from build123d import *

# Parameters (mm, degrees)
CROQUIS1_W              = 76
CROQUIS1_H              = 85
SALIENTE_EXTRUIR1_DEPTH = 5
SALIENTE_EXTRUIR5_DEPTH = 5
CROQUIS6_W              = 76
CROQUIS6_H              = 85
CROQUIS6_W_2            = 68
CROQUIS6_H_2            = 77
SALIENTE_EXTRUIR6_DEPTH = 50
REDONDEO1_R             = 10
CROQUIS7_W              = 15
CROQUIS7_H              = 28
CORTAR_EXTRUIR2_DEPTH   = 5
CROQUIS8_W              = 30
CROQUIS8_H              = 30
CORTAR_EXTRUIR3_DEPTH   = 3
CROQUIS10_W             = 4
CROQUIS10_H             = 4
SALIENTE_EXTRUIR7_DEPTH = 1.5


with BuildPart() as part:
    # Croquis1 → Saliente-Extruir1 (new body)
    with BuildSketch(Plane.XY):
        Rectangle(CROQUIS1_W, CROQUIS1_H)
    extrude(amount=SALIENTE_EXTRUIR1_DEPTH)

    # Croquis5 → Saliente-Extruir5 (add)
    with BuildSketch(Plane.XY.offset(5)):
        Polygon((25.754700538, -30), (22, -30), (22, -34), (34, -34), (34, -22), (30, -22), (30, -25.575128869), (31.4, -28), (29.7, -30.944486373), (26.3, -30.944486373), align=None)
        Polygon((22, -22), (22, -30), (25.754700538, -30), (24.6, -28), (26.3, -25.055513627), (29.7, -25.055513627), (30, -25.575128869), (30, -22), align=None)
        Polygon((-22, -30), (-25.754700538, -30), (-26.3, -30.944486373), (-29.7, -30.944486373), (-31.4, -28), (-30, -25.575128869), (-30, -22), (-34, -22), (-34, -34), (-22, -34), align=None)
        Polygon((-24.6, -28), (-25.754700538, -30), (-22, -30), (-22, -22), (-30, -22), (-30, -25.575128869), (-29.7, -25.055513627), (-26.3, -25.055513627), align=None)
        Polygon((-30, 25.575128869), (-30, 22), (-22, 22), (-22, 30), (-25.754700538, 30), (-24.6, 28), (-26.3, 25.055513627), (-29.7, 25.055513627), align=None)
        Polygon((-34, 22), (-30, 22), (-30, 25.575128869), (-31.4, 28), (-29.7, 30.944486373), (-26.3, 30.944486373), (-25.754700538, 30), (-22, 30), (-22, 34), (-34, 34), align=None)
        Polygon((30, 25.575128869), (30, 22), (34, 22), (34, 34), (22, 34), (22, 30), (25.754700538, 30), (26.3, 30.944486373), (29.7, 30.944486373), (31.4, 28), align=None)
        Polygon((22, 22), (30, 22), (30, 25.575128869), (29.7, 25.055513627), (26.3, 25.055513627), (24.6, 28), (25.754700538, 30), (22, 30), align=None)
    extrude(amount=SALIENTE_EXTRUIR5_DEPTH)

    # Croquis6 → Saliente-Extruir6 (add)
    with BuildSketch(Plane.XY.offset(5)):
        Rectangle(CROQUIS6_W, CROQUIS6_H)
        Rectangle(CROQUIS6_W_2, CROQUIS6_H_2, mode=Mode.SUBTRACT)
    extrude(amount=SALIENTE_EXTRUIR6_DEPTH)

    # Redondeo1
    redondeo1_edges = [part.edges().sort_by_distance(p)[0] for p in [
        (0, 42.5, 0),
        (38, 0, 0),
        (0, -42.5, 0),
        (-38, 0, 0),
        (-38, 42.5, 27.5),
        (38, 42.5, 27.5),
        (38, -42.5, 27.5),
        (-38, -42.5, 27.5),
    ]]
    fillet(redondeo1_edges, radius=REDONDEO1_R)

    # Croquis7 → Cortar-Extruir2 (cut)
    with BuildSketch(Plane(origin=(38, 0, 0), x_dir=(0, 0, -1), z_dir=(1, 0, 0))):
        with Locations((-32.5, 0)):
            Rectangle(CROQUIS7_W, CROQUIS7_H)
    extrude(amount=-CORTAR_EXTRUIR2_DEPTH, mode=Mode.SUBTRACT)

    # Croquis8 → Cortar-Extruir3 (cut)
    with BuildSketch(Plane.ZY.offset(-34)):
        with Locations((34, 0)):
            Rectangle(CROQUIS8_W, CROQUIS8_H)
    extrude(amount=-CORTAR_EXTRUIR3_DEPTH, mode=Mode.SUBTRACT)

    # Croquis10 → Saliente-Extruir7 (add)
    with BuildSketch(Plane.ZY.offset(-37)):
        with Locations((21, -13)):
            Rectangle(CROQUIS10_W, CROQUIS10_H)
        with Locations((47, -13)):
            Rectangle(CROQUIS10_W, CROQUIS10_H)
        with Locations((47, 13)):
            Rectangle(CROQUIS10_W, CROQUIS10_H)
        with Locations((21, 13)):
            Rectangle(CROQUIS10_W, CROQUIS10_H)
    extrude(amount=SALIENTE_EXTRUIR7_DEPTH)


solid = part.part
Geometry check sheet. Reference: the model listing, model coordinates, mm. A direction names the side the tool comes from. Round coordinates to 2 decimals unless told otherwise and drop trailing zeros. Write each loop counter-clockwise with the first axis right and the second up, starting at its lowest first coordinate (ties: lowest second). Pieces come first, ordered by that corner, then holes. Notation, with made-up numbers: (88, 62.5) - (138, 62.5) arc R15 cw to (138, 66.5) - close; hole circle Ø1 at (-9, 11). An arc over 180 degrees is marked (long way). One line per item, written item: value.
1. Cross-section at D-D on y = 20.5. Record the boundary of the cut face in (x, z).
The answers:
outline: (-38, 10) arc R10 ccw to (-28, 0) - (28, 0) arc R10 ccw to (38, 10) - (38, 55) - (34, 55) - (34, 5) - (-34, 5) - (-34, 55) - (-38, 55) - close
2. Scan lines: L1, parallel to Y at x = -10, z = 34.5; L2, parallel to X at y = 24, z = 20; L3, parallel to Z at x = 19.5, y = 10. Record each from-to range of solid material in increasing order.
The answers:
L1: y = -42.5 to -38.5, 38.5 to 42.5
L2: x = -38 to -34, 34 to 38
L3: z = 0 to 5
3. Cross-section at C-C on x = -20. Record the boundary of the cut face in (y, z), and give its area (3 significant figures).
The answers:
outline: (-42.5, 10) arc R10 ccw to (-32.5, 0) - (32.5, 0) arc R10 ccw to (42.5, 10) - (42.5, 55) - (38.5, 55) - (38.5, 5) - (-38.5, 5) - (-38.5, 55) - (-42.5, 55) - close
area: 782 mm^2
4. Cross-section at B-B on z = 13. Record the boundary of the cut face in (x, y), and give its area (3 significant figures).
The answers:
outline: (-38, -32.5) arc R10 ccw to (-28, -42.5) - (28, -42.5) arc R10 ccw to (38, -32.5) - (38, 32.5) arc R10 ccw to (28, 42.5) - (-28, 42.5) arc R10 ccw to (-38, 32.5) - close; hole (-34, -38.5) - (34, -38.5) - (34, 38.5) - (-34, 38.5) - close
area: 1,140 mm^2
5. Set-up check for faces 4 (the face through (30.54, 29.49, 7.46)), 5 (the face through (35.5, 13, 21)), 6 (the face through (-35.15, 0.45, 3.01)): record each of +Z, -Z, +X, -X, +Y, -Y from which the full face is reachable in a straight line by a thin tool's end or side.
The answers:
face 4: +Z
face 5: none
face 6: -Z, -X, +Y, -Y
6. Depth check by flat-ended pin: pin 1 Ø3.5 at (x, z) = (-28, 6.5) entering from +Y; pin 2 Ø2.5 at (x, z) = (-27.5, 6.5) entering from -Y; pin 3 Ø4 at (x, y) = (17, 25.5) entering from +Z. Enter the tip coordinate at first touch or a pass-through.
The answers:
pin 1: stops at y = 42.35
pin 2: stops at y = -42.24
pin 3: stops at z = 5
7. Mould release check, pull along Z, two halves, no side actions. Record for faces 1 (the face through (-28, -34, 7)), 2 (the face through (35.5, 13, 47)), 3 (the face through (-31, 29, 10)): released by +Z, released by -Z, zero draft, split by the parting line, or undercut.
The answers:
face 1: zero draft
face 2: undercut
face 3: released by +Z
8. Cross-section at A-A on y = -4. Record the boundary of the cut face in (x, z).
The answers:
outline: (-38, 10) arc R10 ccw to (-28, 0) - (28, 0) arc R10 ccw to (38, 10) - (38, 25) - (37, 25) - (37, 19) - (34, 19) - (34, 5) - (-34, 5) - (-34, 55) - (-38, 55) - close; (34, 49) - (37, 49) - (37, 40) - (38, 40) - (38, 55) - (34, 55) - close
